Here's how the part is built. I have some questions about the finished solid (model axes, mm). A direction names the side the tool comes from. Round coordinates to 2 decimals unless told otherwise and drop trailing zeros. Loops run counter-clockwise (first coordinate to the right, second up) from the corner with the lowest first, then second, coordinate; pieces in that order, holes last. Notation, with made-up numbers: M 73.5,32.25 L 115.5,32.25 A17 ccw 115.5,42.25 Z; hole C 44.25,43.25 d8. An arc over 180 degrees is marked long. Answer as a JSON object with one key per item and string values.
from build123d import *

# Parameters (mm, degrees)
F2_SIZE = 0.762


with BuildPart() as f1:
    # F0 (on Right) → F1 (revolve)
    with BuildSketch(Plane.YZ):
        Polygon((0, 152.4), (0, 0), (9.525, 0), (9.525, 5.5626), (6.35, 5.5626), (6.35, 13.5001), (9.525, 13.5001), (9.525, 152.4), align=None)
    revolve(axis=Axis((0, 0, 76.2), (0, 0, -1)))

    # F2
    f2_edges = [f1.edges().sort_by_distance(p)[0] for p in [
        (0, -9.525, 152.4),
        (0, -9.525, 5.5626),
        (0, -9.525, 13.5001),
        (0, -9.525, 0),
    ]]
    chamfer(f2_edges, length=F2_SIZE)


solid = f1.part
Item 1: I want a section at C-C on z = 124. List the corners of the cut face in (x, y) for me (3 decimals), plus the area to 3 significant figures.
Solution:
{"outline": "C 0,0 d19.05", "area": "285 mm2"}
Item 2: For P1, Ø5, axis at y = 6, z = 17, coming from the +X side, with a flat end and sliding along its axis, tell me the tip position at first contact or that it passes through.
Solution:
{"P1": "stops at x = 8.86"}
Item 3: We'd pull the mould along Z, two halves only. Please class faces 1 (the face through (3, 6, 5.563)), 2 (the face through (-5.796, -7.559, 83.912)), 3 (the face through (0, 0, 0)), 4 (the face through (0, 0, 152.4)): +Z half, -Z half, draft (parallel to the pull), parting line (faces both ways), or undercut.
Solution:
{"face 1": "undercut", "face 2": "draft", "face 3": "-Z half", "face 4": "+Z half"}
Item 4: I want a section at A-A on y = 0. List the corners of the cut face in (x, z) for me (3 decimals).
Solution:
{"outline": "M -9.525,0.762 L -8.763,0 L 8.763,0 L 9.525,0.762 L 9.525,4.801 L 8.763,5.563 L 6.35,5.563 L 6.35,13.5 L 8.763,13.5 L 9.525,14.262 L 9.525,151.638 L 8.763,152.4 L -8.763,152.4 L -9.525,151.638 L -9.525,14.262 L -8.763,13.5 L -6.35,13.5 L -6.35,5.563 L -8.763,5.563 L -9.525,4.801 Z"}
Item 5: For faces 5 (the face through (-5.796, -7.559, 2.81)), 6 (the face through (3, -6, 13.5)), which set-ups out of +Z, -Z, +X, -X, +Y, -Y let a thin tool reach every point of the face, with its end or its side?
Solution:
{"face 5": "+Z, -Z", "face 6": "none"}
Item 6: If I drill on L1, parallel to Z at x = -3.5, y = 6.75; L2, parallel to Y at x = -3.75, z = 26; L3, parallel to Z at x = -3, y = 8.5, over which ranges is the centre line in solid material (lowest first)? Write a range as from..to.
Solution:
{"L1": "z = 0..5.56, 13.5..152.4", "L2": "y = -8.76..8.76", "L3": "z = 0.25..5.31, 13.75..152.15"}
